For this review, use the dimensioned drawing (mm, ordinates from the lowest corner) and the shaded views. Round coordinates to 2 decimals unless told otherwise and drop trailing zeros. Write each loop counter-clockwise with the first axis right and the second up, starting at its lowest first coordinate (ties: lowest second). Pieces come first, ordered by that corner, then holes. Notation, with made-up numbers: M 35.25,17 L 57.25,17 A20 cw 57.25,56 Z; hole C -15,75.25 d10. An arc over 180 degrees is marked long. Answer in a Markdown table with one row per item.
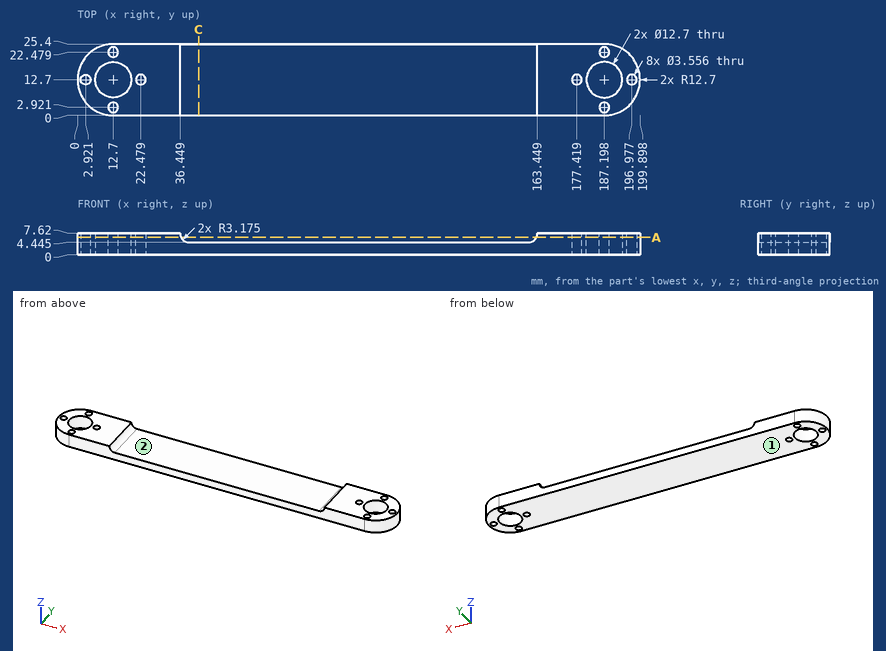
Q1. Take a section at C-C (x = 43). State the section outline as (y, z) points (3 decimals).
Found:
| item | result |
|---|---|
| outline | M 0,0 L 25.4,0 L 25.4,4.445 L 0,4.445 Z |
Q2. Mouldability with a two-part tool opening along X and no side actions: class the marked faces 1 and 2 as +X half, -X half, draft (parallel to the pull), parting line (faces both ways), or undercut.
Found:
| item | result |
|---|---|
| face 1 | draft |
| face 2 | undercut |
Q3. For probe 1 along Y at (x, z) = (12, 1.25); probe 2 along X at (y, z) = (17.75, 2.25); probe 3 along X at (y, z) = (1.5, 2.5) (1 decimal), list the stretches that pass through material, from the lowest coordinate up.
Found:
| item | result |
|---|---|
| probe 1 | 0.02 to 1.29, 4.56 to 6.39, 19.01 to 20.84, 24.11 to 25.38 |
| probe 2 | 1.05 to 8.85, 16.55 to 183.35, 191.05 to 198.85 |
| probe 3 | 6.7 to 11.6, 13.8 to 186.1, 188.3 to 193.2 |
Q4. Take a section at A-A (z = 6.25). State how many separate pieces and enclosed holes the cut face has, then the cut area to 3 significant figures.
Found:
| item | result |
|---|---|
| separate pieces | 2 |
| enclosed holes | 10 |
| area | 1,400 mm² |
Q5. Insertion check: P1, Ø3, axis at y = 14, z = 5.5, coming from the +X side; P2, Ø1.5, axis at x = 121, z = 5.5, coming from the +Y side; P3, Ø3, axis at x = 84.5, y = 12.5, coming from the +Z side (3 decimals); P4, Ø1, axis at y = 5, z = 6, coming from the +X side. Each pin has a flat end and moves straight along its axis. Give the tip position at first contact, or say it passes through.
Found:
| item | result |
|---|---|
| P1 | x = 199.9 |
| P2 | through |
| P3 | z = 4.445 |
| P4 | x = 197.66 |
